Verification items for the finished model (mm, model axes). A direction names the side the tool comes from. Round coordinates to 2 decimals unless told otherwise and drop trailing zeros. Loops run counter-clockwise (first coordinate to the right, second up) from the corner with the lowest first, then second, coordinate; pieces in that order, holes last. Notation, with made-up numbers: (0, 84.25) -> (19, 84.25) arc R11 cw to (19, 102.25) -> close; hole circle Ø2 at (8.5, 58.5). An arc over 180 degrees is marked (long way). Write item = value, one per line. Start each with the question number.
```python
from build123d import *

# Parameters (mm, degrees)
ESQUISSE5_W             = 255.35
ESQUISSE5_H             = 22
BOSS_EXTRU_1_DEPTH      = 10
ESQUISSE6_R             = 3
ENL_V_MAT_EXTRU_4_DEPTH = 173.494473459
ESQUISSE7_W             = 22
ESQUISSE7_H             = 22
ENL_V_MAT_EXTRU_5_DEPTH = 5


with BuildPart() as part:
    # Esquisse5 → Boss.-Extru.1 (new body)
    with BuildSketch(Plane.XY):
        with Locations((41.235968465, 22.517579062)):
            Rectangle(ESQUISSE5_W, ESQUISSE5_H)
    extrude(amount=BOSS_EXTRU_1_DEPTH)

    # Esquisse6 → Enlèv. mat.-Extru.4 (cut, through all)
    with BuildSketch(Plane.XY):
        with Locations((-75.439031535, 22.517579062)):
            Circle(ESQUISSE6_R)
        with Locations((157.910968465, 22.517579062)):
            Circle(ESQUISSE6_R)
    extrude(amount=ENL_V_MAT_EXTRU_4_DEPTH, mode=Mode.SUBTRACT)

    # Esquisse7 → Enlèv. mat.-Extru.5 (cut)
    with BuildSketch(Plane.XY.offset(10)):
        with Locations((-75.439031535, 22.517579062)):
            Rectangle(ESQUISSE7_W, ESQUISSE7_H)
        with Locations((157.910968465, 22.517579062)):
            Rectangle(ESQUISSE7_W, ESQUISSE7_H)
    extrude(amount=-ENL_V_MAT_EXTRU_5_DEPTH, mode=Mode.SUBTRACT)


solid = part.part
```
(1) Section check B-B on z = 6.5. Enter the section's corners in (x, y), then the cut area to 3 significant figures.
(2) Depth check by flat-ended pin: pin 1 Ø2.5 at (y, z) = (26, 7.5) entering from -X; pin 2 Ø6.5 at (x, y) = (-78.5, 19) entering from +Z. Enter the tip coordinate at first touch or a pass-through.
(3) Scan lines: line 1 (X direction, y = 20.5, z = 1.75); line 2 (Z direction, x = -75.5, y = 15.5); line 3 (X direction, y = 21.75, z = 6). Record each from-to range of solid material in increasing order. Write a range as [from, to].
(4) Draft check along X on faces 4 (the flat face through (39, 33.518, 5)), 5 (the flat face through (168.911, 22, 2)), 6 (the cylindrical face through (154.914, 22.649, 2.465)). Enter one of: +X half, -X half, draft (parallel to the pull), parting line (faces both ways), or undercut.
(5) Access from +Z, -Z, +X, -X, +Y, -Y to the whole of each face (thin tool, end or side, straight path). Record for faces 1 (the flat face through (146.911, 22, 8)), 2 (the flat face through (-78, 20, 5)), 3 (the flat face through (39, 11.518, 5)).
(6) Section check A-A on y = 30. Enter the section's corners in (x, z), then the cut area to 3 significant figures.
Computed values:
q1.outline = (-64.44, 11.52) -> (146.91, 11.52) -> (146.91, 33.52) -> (-64.44, 33.52) -> close
q1.area = 4,650 mm²
q2.pin_1 = -64.44
q2.pin_2 = 5
q3.line_1 = [-86.44, -77.66], [-73.22, 155.69], [160.13, 168.91]
q3.line_2 = [0, 5]
q3.line_3 = [-64.44, 146.91]
q4.face_4 = draft
q4.face_5 = +X half
q4.face_6 = undercut
q5.face_1 = +Z, +X, +Y, -Y
q5.face_2 = +Z, -X, +Y, -Y
q5.face_3 = +Z, -Z, +X, -X, -Y
q6.outline = (-86.44, 0) -> (168.91, 0) -> (168.91, 5) -> (146.91, 5) -> (146.91, 10) -> (-64.44, 10) -> (-64.44, 5) -> (-86.44, 5) -> close
q6.area = 2,330 mm²
